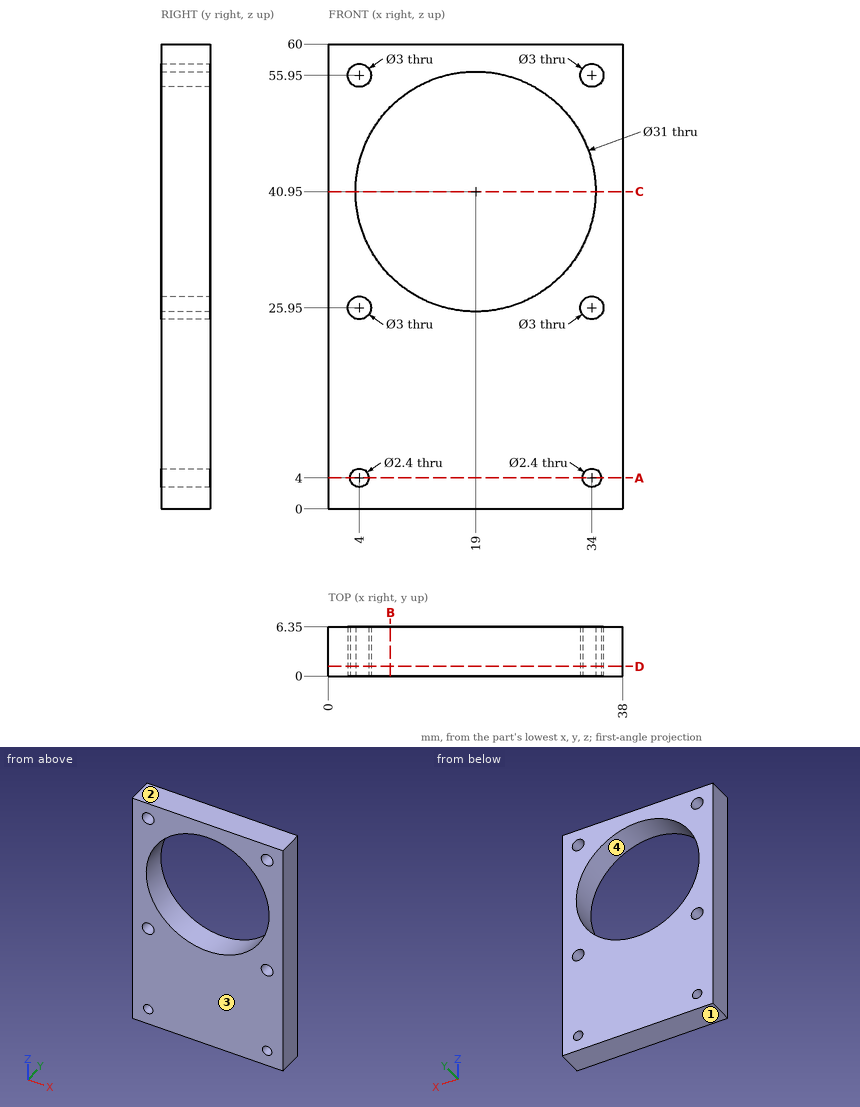
Study the drawing (mm; zero at the part's minimum x, y, z) and answer. Coordinates: 2 decimals unless noted, no trailing zeros. Write each loop counter-clockwise with the first axis right and the second up, starting at its lowest first coordinate (ties: lowest second). Pieces come first, ordered by that corner, then holes. Notation, with made-up numbers: (32.25, 17.5) -> (80.25, 17.5) arc R29 cw to (80.25, 39.5) -> close; hole circle Ø11 at (87.5, -15.75). An arc over 180 degrees is marked (long way). Write item = value, one per line.
(1) Straight lines are drawn through the part: L1, parallel to X at y = 5, z = 27; L2, parallel to X at y = 5, z = 30.5; L3, parallel to Z at x = 16.5, y = 3. For each, find the intervals that lie inside material, in ascending order. Write a range as from..to.
From the geometry:
L1 = 0..2.93, 5.07..12.24, 25.76..32.93, 35.07..38
L2 = 0..7.55, 30.45..38
L3 = 0..25.65, 56.25..60
(2) Section D-D on y = 1.25 is taken. Write down the section's boundary in (x, z), plus the area to 3 significant figures.
From the geometry:
outline = (0, 0) -> (38, 0) -> (38, 60) -> (0, 60) -> close; hole circle Ø3 at (4, 25.95); hole circle Ø3 at (4, 55.95); hole circle Ø2.4 at (4, 4); hole circle Ø31 at (19, 40.95); hole circle Ø3 at (34, 25.95); hole circle Ø3 at (34, 55.95); hole circle Ø2.4 at (34, 4)
area = 1,490 mm2
(3) Section A-A on z = 4 is taken. Write down the section's boundary in (x, y).
From the geometry:
outline = (0, 0) -> (2.8, 0) -> (2.8, 6.35) -> (0, 6.35) -> close; (5.2, 0) -> (32.8, 0) -> (32.8, 6.35) -> (5.2, 6.35) -> close; (35.2, 0) -> (38, 0) -> (38, 6.35) -> (35.2, 6.35) -> close
(4) For a pull along Z with two mould halves and no side action, classify the marked faces 1, 2, 3 and 4 as +Z half, -Z half, draft (parallel to the pull), parting line (faces both ways), or undercut.
From the geometry:
face_1 = -Z half
face_2 = +Z half
face_3 = draft
face_4 = undercut
(5) Section B-B on x = 8 is taken. Write down the section's boundary in (y, z).
From the geometry:
outline = (0, 0) -> (6.35, 0) -> (6.35, 30.03) -> (0, 30.03) -> close; (0, 51.87) -> (6.35, 51.87) -> (6.35, 60) -> (0, 60) -> close
(6) Section C-C on z = 40.95 is taken. Write down the section's boundary in (x, y), plus the area to 4 significant figures.
From the geometry:
outline = (0, 0) -> (3.5, 0) -> (3.5, 6.35) -> (0, 6.35) -> close; (34.5, 0) -> (38, 0) -> (38, 6.35) -> (34.5, 6.35) -> close
area = 44.45 mm2
